from build123d import *

# Parameters (mm, degrees)
SKETCH1_W                                      = 82.55
SKETCH1_H                                      = 31.75
PLATE_DEPTH                                    = 1.5875
F_10_CLEARANCE_HOLE1_D                         = 5.1054
CBORE_FOR_4_SOCKET_HEAD_CAP_SCREW1_D           = 3.2639
CBORE_FOR_4_SOCKET_HEAD_CAP_SCREW1_CBORE_D     = 5.55752
CBORE_FOR_4_SOCKET_HEAD_CAP_SCREW1_CBORE_DEPTH = 9.1948


with BuildPart() as part:
    # Sketch1 → Plate (new, symmetric)
    with BuildSketch(Plane(origin=(0, 0, 0), x_dir=(1, 0, 0), z_dir=(0, 1, 0))):
        Rectangle(SKETCH1_W, SKETCH1_H)
    extrude(amount=PLATE_DEPTH, both=True)

    # #10 Clearance Hole1 (through all)
    with Locations(Plane(origin=(0, 1.5875, 0), x_dir=(1, 0, 0), z_dir=(0, 1, 0))):
        with Locations((-36.5125, 11.1125), (36.5125, 11.1125), (36.5125, -11.1125), (-36.5125, -11.1125), (0, -11.1125), (0, 11.1125)):
            Hole(F_10_CLEARANCE_HOLE1_D / 2)

    # CBORE for #4 Socket Head Cap Screw1 (through all)
    with Locations(Plane(origin=(0, 1.5875, 0), x_dir=(1, 0, 0), z_dir=(0, 1, 0))):
        with Locations((0, 0), (36.5125, 0), (18.25625, 11.1125), (18.25625, -11.1125)):
            CounterBoreHole(CBORE_FOR_4_SOCKET_HEAD_CAP_SCREW1_D / 2, CBORE_FOR_4_SOCKET_HEAD_CAP_SCREW1_CBORE_D / 2, CBORE_FOR_4_SOCKET_HEAD_CAP_SCREW1_CBORE_DEPTH)


solid = part.part
The listing builds one solid part. Answer for the finished solid, in the listing's coordinates (mm). Round coordinates to 2 decimals unless told otherwise and drop trailing zeros. Order: outer loops, then holes, each group sorted by start corner. A loop starts at its lowest first (then second) coordinate and runs counter-clockwise, first axis right, second up. Notation, with made-up numbers: M -33,34.5 L 14,34.5 A21 ccw 14,61.5 Z; hole C 83.25,54 d9. An arc over 180 degrees is marked long. Answer in a Markdown table with one row per item. Add a question column.
1) The part is cut by section B-B on z = 0. Determine the outline of the cut face in (x, y) (1 decimal), plus the area to 3 significant figures.
2) The part is cut by section A-A on x = 0. Determine the outline of the cut face in (y, z) (1 decimal).
3) The part is cut by section D-D on z = -9.5. Determine the outline of the cut face in (x, y) (1 decimal).
4) Determine the mould class of faces 1 (the face through (0.553, -0.022, 13.604)), 2 (the face through (19.75, 0.022, -13.456)), 3 (the face through (41.275, 0, 0)), 4 (the face through (-1, 0, 15.875)) for opening direction Z: pulls with the +Z half, pulls with the -Z half, needs draft (parallel to the pull), parting line crosses it, or undercut.
5) Consider line 1 along X through (y, z) = (0.6, 11) (3 decimals); line 2 along Z through (x, y) = (0, -0.3) (3 decimals); line 3 along Z through (x, y) = (-36, -0.65) (3 decimals). Determine where each line is inside the solid, lowest interval first. Write a range as from..to.
6) A flat-ended cylindrical pin translates along its axis: pin 1 Ø3 at (x, z) = (0, 11.11) entering from -Y. Find the tip coordinate at first contact, or state that the pin passes through.
7) The part is cut by section C-C on y = 0.8. Count the separate pieces of the cut face and the enclosed holes in it, plus the area to 3 significant figures.
Findings below:
| question | item | result |
|---|---|---|
| 1 | outline | M -41.3,-1.6 L -2.8,-1.6 L -2.8,1.6 L -41.3,1.6 Z; M 2.8,-1.6 L 33.7,-1.6 L 33.7,1.6 L 2.8,1.6 Z; M 39.3,-1.6 L 41.3,-1.6 L 41.3,1.6 L 39.3,1.6 Z |
| 1 | area | 227 mm² |
| 2 | outline | M -1.6,-15.9 L 1.6,-15.9 L 1.6,-13.7 L -1.6,-13.7 Z; M -1.6,-8.6 L 1.6,-8.6 L 1.6,-2.8 L -1.6,-2.8 Z; M -1.6,2.8 L 1.6,2.8 L 1.6,8.6 L -1.6,8.6 Z; M -1.6,13.7 L 1.6,13.7 L 1.6,15.9 L -1.6,15.9 Z |
| 3 | outline | M -41.3,-1.6 L -38.5,-1.6 L -38.5,1.6 L -41.3,1.6 Z; M -34.5,-1.6 L -2,-1.6 L -2,1.6 L -34.5,1.6 Z; M 2,-1.6 L 16,-1.6 L 16,1.6 L 2,1.6 Z; M 20.5,-1.6 L 34.5,-1.6 L 34.5,1.6 L 20.5,1.6 Z; M 38.5,-1.6 L 41.3,-1.6 L 41.3,1.6 L 38.5,1.6 Z |
| 4 | face 1 | undercut |
| 4 | face 2 | undercut |
| 4 | face 3 | needs draft |
| 4 | face 4 | pulls with the +Z half |
| 5 | line 1 | x = -41.275..-39.063, -33.962..-2.55, 2.55..15.48, 21.033..33.962, 39.063..41.275 |
| 5 | line 2 | z = -15.875..-13.665, -8.56..-2.779, 2.779..8.56, 13.665..15.875 |
| 5 | line 3 | z = -15.875..-13.613, -8.612..8.612, 13.613..15.875 |
| 6 | pin 1 | passes through |
| 7 | separate pieces | 1 |
| 7 | enclosed holes | 10 |
| 7 | area | 2,400 mm² |
